Geometry: final body of the model. Coordinates: model frame, mm. Face numbers are marked on the shaded views. A direction names the side the tool comes from. Give positions to 0.01 mm unless a question says otherwise; leave off trailing zeros. Loops run counter-clockwise (first coordinate to the right, second up) from the corner with the lowest first, then second, coordinate; pieces in that order, holes last.
from build123d import *

# Parameters (mm, degrees)
SKETCH1_R           = 22.5
SKETCH1_R_2         = 20.9
BOSS_EXTRUDE1_DEPTH = 44
SKETCH1_2_R         = 20.9
BOSS_EXTRUDE2_DEPTH = 111
SKETCH3_R           = 5.025
CUT_EXTRUDE1_DEPTH  = 171
SKETCH2_R           = 13
BOSS_EXTRUDE5_DEPTH = 2
SKETCH2_4_R         = 5
CUT_EXTRUDE2_DEPTH  = 35
SKETCH6_R           = 1.5
CUT_EXTRUDE4_DEPTH  = 10
SKETCH6_3_R         = 1.5
CUT_EXTRUDE5_DEPTH  = 10
SKETCH6_4_R         = 1.5
CUT_EXTRUDE6_DEPTH  = 10
SKETCH6_5_R         = 1.5
CUT_EXTRUDE7_DEPTH  = 10
SKETCH6_7_R         = 4.5
CUT_EXTRUDE8_DEPTH  = 4
SKETCH6_8_R         = 4.5
CUT_EXTRUDE9_DEPTH  = 4
SKETCH6_9_R         = 4.5
CUT_EXTRUDE10_DEPTH = 4
SKETCH6_10_R        = 4.5
CUT_EXTRUDE11_DEPTH = 4


with BuildPart() as part:
    # Sketch1 → Boss-Extrude1 (new body)
    with BuildSketch(Plane.XY):
        Circle(SKETCH1_R)
        Circle(SKETCH1_R_2, mode=Mode.SUBTRACT)
    extrude(amount=BOSS_EXTRUDE1_DEPTH)

    # Sketch1<2> → Boss-Extrude2 (add)
    with BuildSketch(Plane.XY):
        Circle(SKETCH1_2_R)
    extrude(amount=BOSS_EXTRUDE2_DEPTH)

    # Sketch3 → Cut-Extrude1 (cut)
    with BuildSketch(Plane(origin=(0, 0, 0), x_dir=(-1, 0, 0), z_dir=(0, 0, -1))):
        Circle(SKETCH3_R)
    extrude(amount=-CUT_EXTRUDE1_DEPTH, mode=Mode.SUBTRACT)

    # Sketch2 → Boss-Extrude5 (add)
    with BuildSketch(Plane(origin=(0, 0, 0), x_dir=(-1, 0, 0), z_dir=(0, 0, -1))):
        Circle(SKETCH2_R)
    extrude(amount=BOSS_EXTRUDE5_DEPTH)

    # Sketch2<4> → Cut-Extrude2 (cut)
    with BuildSketch(Plane(origin=(0, 0, 0), x_dir=(-1, 0, 0), z_dir=(0, 0, -1))):
        Circle(SKETCH2_4_R)
    extrude(amount=CUT_EXTRUDE2_DEPTH, mode=Mode.SUBTRACT)

    # Sketch6 → Cut-Extrude4 (cut)
    with BuildSketch(Plane(origin=(0, 0, -2), x_dir=(-1, 0, 0), z_dir=(0, 0, -1))):
        with Locations((0, 17.5)):
            Circle(SKETCH6_R)
    extrude(amount=-CUT_EXTRUDE4_DEPTH, mode=Mode.SUBTRACT)

    # Sketch6<3> → Cut-Extrude5 (cut)
    with BuildSketch(Plane(origin=(0, 0, -2), x_dir=(-1, 0, 0), z_dir=(0, 0, -1))):
        with Locations((17.5, 0)):
            Circle(SKETCH6_3_R)
    extrude(amount=-CUT_EXTRUDE5_DEPTH, mode=Mode.SUBTRACT)

    # Sketch6<4> → Cut-Extrude6 (cut)
    with BuildSketch(Plane(origin=(0, 0, -2), x_dir=(-1, 0, 0), z_dir=(0, 0, -1))):
        with Locations((0, -17.5)):
            Circle(SKETCH6_4_R)
    extrude(amount=-CUT_EXTRUDE6_DEPTH, mode=Mode.SUBTRACT)

    # Sketch6<5> → Cut-Extrude7 (cut)
    with BuildSketch(Plane(origin=(0, 0, -2), x_dir=(-1, 0, 0), z_dir=(0, 0, -1))):
        with Locations((-17.5, 0)):
            Circle(SKETCH6_5_R)
    extrude(amount=-CUT_EXTRUDE7_DEPTH, mode=Mode.SUBTRACT)

    # Sketch6<7> → Cut-Extrude8 (cut)
    with BuildSketch(Plane(origin=(0, 0, -2), x_dir=(-1, 0, 0), z_dir=(0, 0, -1))):
        with Locations((12.374368671, 12.374368671)):
            Circle(SKETCH6_7_R)
    extrude(amount=-CUT_EXTRUDE8_DEPTH, mode=Mode.SUBTRACT)

    # Sketch6<8> → Cut-Extrude9 (cut)
    with BuildSketch(Plane(origin=(0, 0, -2), x_dir=(-1, 0, 0), z_dir=(0, 0, -1))):
        with Locations((-12.374368671, 12.374368671)):
            Circle(SKETCH6_8_R)
    extrude(amount=-CUT_EXTRUDE9_DEPTH, mode=Mode.SUBTRACT)

    # Sketch6<9> → Cut-Extrude10 (cut)
    with BuildSketch(Plane(origin=(0, 0, -2), x_dir=(-1, 0, 0), z_dir=(0, 0, -1))):
        with Locations((-12.374368671, -12.374368671)):
            Circle(SKETCH6_9_R)
    extrude(amount=-CUT_EXTRUDE10_DEPTH, mode=Mode.SUBTRACT)

    # Sketch6<10> → Cut-Extrude11 (cut)
    with BuildSketch(Plane(origin=(0, 0, -2), x_dir=(-1, 0, 0), z_dir=(0, 0, -1))):
        with Locations((12.374368671, -12.374368671)):
            Circle(SKETCH6_10_R)
    extrude(amount=-CUT_EXTRUDE11_DEPTH, mode=Mode.SUBTRACT)


solid = part.part
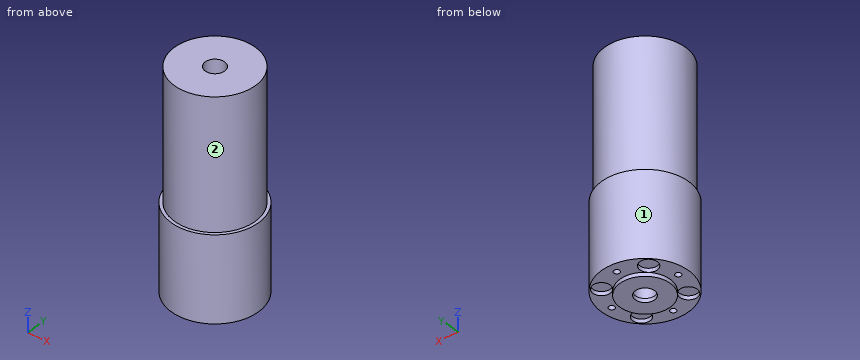
Item 1: Section query A-A on x = 0. Return loops of the section in (y, z) (3 decimals).
Values follow:
outline: (-22.5, 0) - (-19, 0) - (-19, 8) - (-16, 8) - (-16, 0) - (-13, 0) - (-13, -2) - (-5, -2) - (-5, 0) - (-5.025, 0) - (-5.025, 111) - (-20.9, 111) - (-20.9, 44) - (-22.5, 44) - close; (5, -2) - (13, -2) - (13, 0) - (16, 0) - (16, 8) - (19, 8) - (19, 0) - (22.5, 0) - (22.5, 44) - (20.9, 44) - (20.9, 111) - (5.025, 111) - (5.025, 0) - (5, 0) - close
Item 2: Pin query (flat end, axial travel): pin 1 (1.8 mm diameter, centred on x = 0, y = 17.5, fed in from -Z); pin 2 (4.5 mm diameter, centred on x = 14, y = -14, fed in from -Z); pin 3 (10 mm diameter, centred on x = -13, z = 65, fed in from +Y). Return the tip coordinate at first contact, or that it passes through.
Values follow:
pin 1: stops at z = 8
pin 2: stops at z = 0
pin 3: stops at y = 19.31
Item 3: Set-up query: the marked faces 1 and 2. Return all of +Z, -Z, +X, -X, +Y, -Y with unobstructed straight access to the full face (end or side cutting, diameter ignored); none if empty.
Values follow:
face 1: +Z, -Z
face 2: +Z
Item 4: Section query C-C on z = 46.5. Return loops of the section in (x, y) (3 decimals).
Values follow:
outline: circle Ø41.8 at (0, 0); hole circle Ø10.05 at (0, 0)
Item 5: Ray query, probe 1 along Y at (x, z) = (0, 43.5) (3 decimals); probe 2 along Y at (x, z) = (0, 46) (3 decimals); probe 3 along Z at (x, y) = (-10, -17.5). Return the intervals inside material, ascending.
Values follow:
probe 1: y = -22.5 to -5.025, 5.025 to 22.5
probe 2: y = -20.9 to -5.025, 5.025 to 20.9
probe 3: z = 0 to 111
Item 6: Section query D-D on z = 31. Return loops of the section in (x, y) (3 decimals).
Values follow:
outline: circle Ø45 at (0, 0); hole circle Ø10.05 at (0, 0)
